```python
from build123d import *

# Parameters (mm, degrees)
F0_W     = 2575
F0_H     = 40
F1_DEPTH = 628
F2_W     = 2575
F2_H     = 140
F3_DEPTH = 25
F4_W     = 653
F4_H     = 140
F5_DEPTH = 25


with BuildPart() as f1:
    # F0 (on Front) → F1 (new body)
    with BuildSketch(Plane.XZ):
        Rectangle(F0_W, F0_H)
    extrude(amount=F1_DEPTH)

    # F2 (on face) → F3 (join)
    with BuildSketch(Plane(origin=(0, 0, 0), x_dir=(-1, 0, 0), z_dir=(0, 1, 0))):
        with Locations((0, 50)):
            Rectangle(F2_W, F2_H)
    extrude(amount=F3_DEPTH)

    # F4 (on face) → F5 (join)
    with BuildSketch(Plane.YZ.offset(1287.5)):
        with Locations((-301.5, 50)):
            Rectangle(F4_W, F4_H)
    extrude(amount=F5_DEPTH)


solid = f1.part
```
Geometry check sheet. Reference: the model listing, model coordinates, mm. A direction names the side the tool comes from. Coordinates: 2 decimals unless noted, no trailing zeros. Loops run counter-clockwise (first coordinate to the right, second up) from the corner with the lowest first, then second, coordinate; pieces in that order, holes last. Notation, with made-up numbers: (65, -14.75) - (111, -14.75) arc R10 ccw to (111, -6.75) - close; hole circle Ø10 at (-7, -2). An arc over 180 degrees is marked (long way). One line per item, written item: value. Start each with the question number.
(1) Cross-section at B-B on x = -200.5. Enter the section's corners in (y, z).
(2) Depth check by flat-ended pin: P1, Ø12, axis at x = -628, y = -157.5, coming from the +Z side; P2, Ø1, axis at x = -390, z = 31.5, coming from the -Y side. Enter the tip coordinate at first touch or a pass-through.
(3) Tool access check on faces 1 (the flat face through (-6, 25, 49)), 2 (the flat face through (18, 0, 71)). Record the directions out of +Z, -Z, +X, -X, +Y, -Y that give a thin tool (end or side, any length) a straight path to the whole face; none if there is none.
(4) Material ranges on line 1 (X direction, y = -378.5, z = 52); line 2 (Z direction, x = 200, y = -63.5); line 3 (Y direction, x = 951, z = 35), recorded low to high. Write a range as [from, to].
(5) Cross-section at A-A on z = 80.5. Enter the section's corners in (x, y).
Results below:
1. outline: (-628, -20) - (25, -20) - (25, 120) - (0, 120) - (0, 20) - (-628, 20) - close
2. P1: stops at z = 20
2. P2: stops at y = 0
3. face 1: +Z, -Z, +X, -X, +Y
3. face 2: +Z, -X, -Y
4. line 1: x = [1287.5, 1312.5]
4. line 2: z = [-20, 20]
4. line 3: y = [0, 25]
5. outline: (-1287.5, 0) - (1287.5, 0) - (1287.5, -628) - (1312.5, -628) - (1312.5, 25) - (-1287.5, 25) - close
